from build123d import *

# Parameters (mm, degrees)
SKETCH2_R               = 75
SKETCH2_R_2             = 26
BOSS_EXTRUDE1_DEPTH     = 55
CUT_EXTRUDE1_DEPTH      = 120.478031453
CUT_EXTRUDE1_DEPTH_BACK = 52
SKETCH3_R               = 75
FILLET1_R               = 3
CHAMFER1_SIZE           = 2
CHAMFER3_SIZE           = 2
FILLET2_R               = 1


with BuildPart() as part:
    # Sketch2 → Boss-Extrude1 (new body)
    with BuildSketch(Plane(origin=(0, 0, 0), x_dir=(1, 0, 0), z_dir=(0, 1, 0))):
        with Locations(Location((0, 0, 0), (0, 0, 270))):
            Circle(SKETCH2_R)
        with Locations(Location((0, 0, 0), (0, 0, 270))):
            Circle(SKETCH2_R_2, mode=Mode.SUBTRACT)
    extrude(amount=BOSS_EXTRUDE1_DEPTH)

    # Sketch3 → Cut-Extrude1 (cut, two sides: drawn at the far end of the back side and taken through both)
    with BuildSketch(Plane.XZ.offset(-CUT_EXTRUDE1_DEPTH_BACK)):
        with Locations(Location((0, 0, 0), (0, 0, 90))):
            Circle(SKETCH3_R)
        Polygon((32.5, -18.763883749), (32.5, 18.763883749), (0, 37.527767497), (-32.5, 18.763883749), (-32.5, -18.763883749), (0, -37.527767497), align=None, mode=Mode.SUBTRACT)
    extrude(amount=CUT_EXTRUDE1_DEPTH + CUT_EXTRUDE1_DEPTH_BACK, mode=Mode.SUBTRACT)

    # Fillet1
    fillet1_edges = [part.edges().sort_by_distance(p)[0] for p in [
        (0, 26, -37.527767497),
        (-32.5, 26, -18.763883749),
        (-32.5, 26, 18.763883749),
        (0, 26, 37.527767497),
        (32.5, 26, 18.763883749),
        (32.5, 26, -18.763883749),
    ]]
    fillet(fillet1_edges, radius=FILLET1_R)

    # Chamfer1
    chamfer1_edges = [part.edges().sort_by_distance(p)[0] for p in [
        (16.25, 0, -28.145825623),
        (32.5, 0, 0),
        (16.25, 0, 28.145825623),
        (-16.25, 0, 28.145825623),
        (-32.5, 0, 0),
        (-16.25, 0, -28.145825623),
        (0, 0, -37.063665882),
        (-32.098076211, 0, -18.531832941),
        (-32.098076211, 0, 18.531832941),
        (0, 0, 37.063665882),
        (32.098076211, 0, 18.531832941),
        (32.098076211, 0, -18.531832941),
    ]]
    chamfer(chamfer1_edges, length=CHAMFER1_SIZE)

    # Chamfer3
    chamfer3_edges = [part.edges().sort_by_distance(p)[0] for p in [
        (0, 55, -26),
    ]]
    chamfer(chamfer3_edges, length=CHAMFER3_SIZE)

    # Fillet2
    fillet2_edges = [part.edges().sort_by_distance(p)[0] for p in [
        (0, 52, -75),
        (0, 55, -75),
    ]]
    fillet(fillet2_edges, radius=FILLET2_R)


solid = part.part
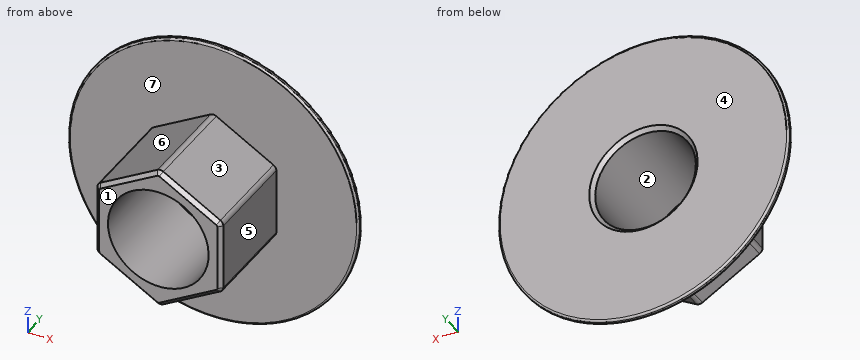
Source: CAD feature listing. Evaluate the final solid. Frame: model axes, mm. Face numbers are marked on the shaded views. A direction names the side the tool comes from. Coordinates: 2 decimals unless noted, no trailing zeros. Loops run counter-clockwise (first coordinate to the right, second up) from the corner with the lowest first, then second, coordinate; pieces in that order, holes last. Notation, with made-up numbers: (51, -21.75) - (68, -21.75) arc R10 cw to (68, -15.75) - close; hole circle Ø5 at (42.25, 29). An arc over 180 degrees is marked (long way). One line per item, written item: value. Start each with the question number.
1. Section A-A (y = 18). Return the cut outline in (x, z), and give its area (3 significant figures).
2. Section B-B (z = 0). Return the cut outline in (x, y), and give its area (3 significant figures).
3. Ray query, L1, parallel to X at y = 41.5, z = 0; L2, parallel to Y at x = 26.5, z = -28; L3, parallel to Z at x = 21.5, y = 32.5. Return the intervals inside material, ascending.
4. Set-up query: the marked faces 4, 5, 6 and 7. Return all of +Z, -Z, +X, -X, +Y, -Y with unobstructed straight access to the full face (end or side cutting, diameter ignored); none if empty.
5. Contact query for flat-ended pins moving along their axis: P1, Ø2, axis at x = -30.5, y = 8.5, coming from the -Z side; P2, Ø2, axis at x = 16.5, y = 23, coming from the -Z side; P3, Ø17, axis at y = 18, z = 1, coming from the +X side. Output: stop coordinate, or through.
6. Mould query, pull axis Z, two halves, no side actions, for the marked faces 1, 2 and 3. Classes: pulls with the +Z half, pulls with the -Z half, needs draft (parallel to the pull), parting line crosses it, or undercut.
Verdict:
1. outline: (-32.5, -17.03) arc R3 ccw to (-31, -19.63) - (-1.5, -36.66) arc R3 ccw to (1.5, -36.66) - (31, -19.63) arc R3 ccw to (32.5, -17.03) - (32.5, 17.03) arc R3 ccw to (31, 19.63) - (1.5, 36.66) arc R3 ccw to (-1.5, 36.66) - (-31, 19.63) arc R3 ccw to (-32.5, 17.03) - close; hole circle Ø52 at (0, 0)
1. area: 1,530 mm2
2. outline: (-75, 53) arc R1 ccw to (-74, 52) - (-32.5, 52) - (-32.5, 2) - (-30.5, 0) - (-26, 0) - (-26, 53) - (-28, 55) - (-74, 55) arc R1 ccw to (-75, 54) - close; (26, 0) - (30.5, 0) - (32.5, 2) - (32.5, 52) - (74, 52) arc R1 ccw to (75, 53) - (75, 54) arc R1 ccw to (74, 55) - (28, 55) - (26, 53) - close
2. area: 961 mm2
3. L1: x = -32.5 to -26, 26 to 32.5
3. L2: y = 52 to 55
3. L3: z = -25.11 to -14.62, 14.62 to 25.11
4. face 4: +Z, -Z, +X, -X, +Y
4. face 5: +Z, -Z, +X, -Y
4. face 6: +Z, -X, -Y
4. face 7: -Y
5. P1: stops at z = -20.5
5. P2: stops at z = -28.58
5. P3: stops at x = 32.5
6. face 1: needs draft
6. face 2: undercut
6. face 3: pulls with the +Z half
